Could you check a few things on this drawing? It's one solid part, dimensions in mm from its lowest x, y, z. A direction names the side the tool comes from. Give positions to 0.01 mm unless a question says otherwise; leave off trailing zeros. Order: outer loops, then holes, each group sorted by start corner. A loop starts at its lowest first (then second) coordinate and runs counter-clockwise, first axis right, second up. Notation, with made-up numbers: (80, 2) -> (127, 2) arc R27 ccw to (127, 34) -> close; hole circle Ø5 at (21.5, -6.5). An arc over 180 degrees is marked (long way). Answer as a JSON object with one key per item and string values.
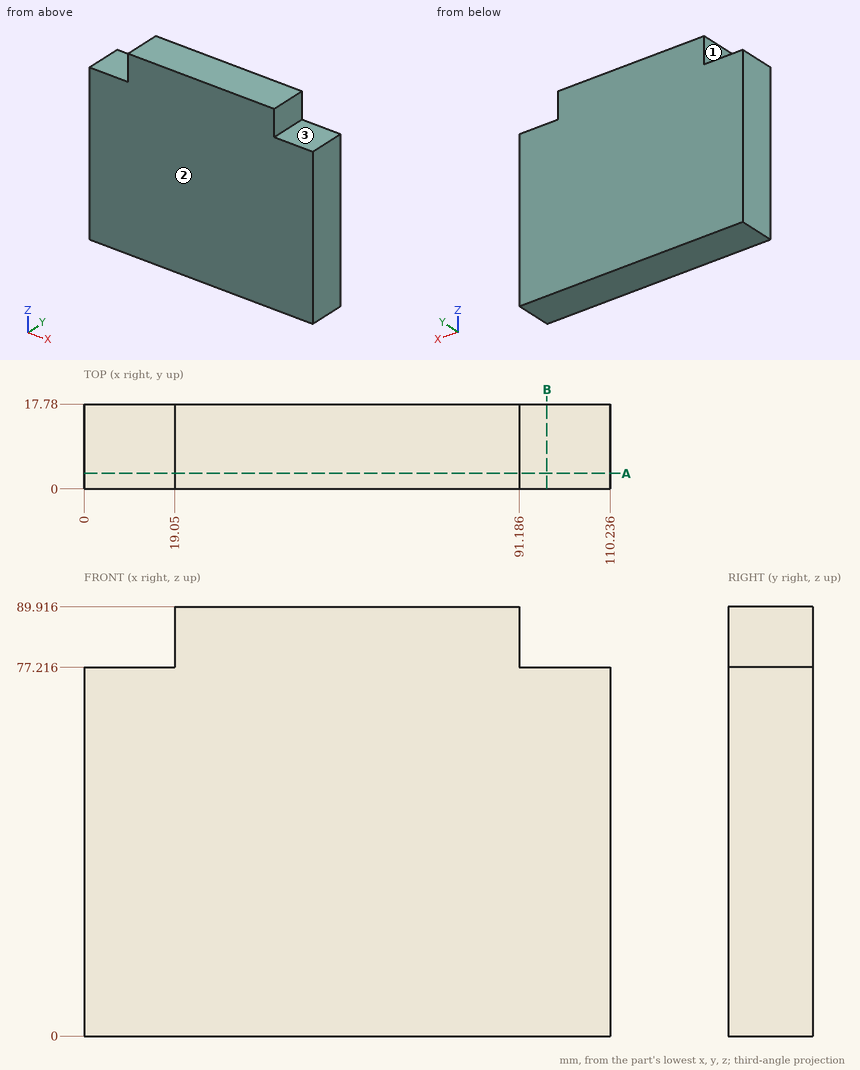
1. For the marked faces 1, 2 and 3, which set-ups out of +Z, -Z, +X, -X, +Y, -Y let a thin tool reach every point of the face, with its end or its side?
Worked answers:
{"face 1": "+Z, -X, +Y, -Y", "face 2": "+Z, -Z, +X, -X, -Y", "face 3": "+Z, +X, +Y, -Y"}
2. If we section it at A-A on y = 3.25: Please give me the cut outline in (x, z), then the cut area to 3 significant figures.
Worked answers:
{"outline": "(0, 0) -> (110.24, 0) -> (110.24, 77.22) -> (91.19, 77.22) -> (91.19, 89.92) -> (19.05, 89.92) -> (19.05, 77.22) -> (0, 77.22) -> close", "area": "9,430 mm²"}
3. Please list where these lines run through material, in increasing order: L1, parallel to Z at x = 101.5, y = 14.75; L2, parallel to X at y = 5.25, z = 84.
Worked answers:
{"L1": "0 to 77.22", "L2": "19.05 to 91.19"}
4. Will these pins go through, and if not, where does the flat tip stop? pin 1 Ø5.5 at (x, y) = (98, 7) entering from +Z; pin 2 Ø4 at (y, z) = (8, 86.5) entering from -X.
Worked answers:
{"pin 1": "z = 77.22", "pin 2": "x = 19.05"}
5. If we section it at B-B on x = 97: Please give me the cut outline in (y, z), then the cut area to 3 significant figures.
Worked answers:
{"outline": "(0, 0) -> (17.78, 0) -> (17.78, 77.22) -> (0, 77.22) -> close", "area": "1,370 mm²"}
